Input: part model. Units: mm. Frame: model coordinates. A direction names the side the tool comes from. Coordinates: 2 decimals unless noted, no trailing zeros. Loops run counter-clockwise (first coordinate to the right, second up) from the corner with the lowest first, then second, coordinate; pieces in that order, holes last. Notation, with made-up numbers: M 80,40 L 119,40 A17 cw 119,71 Z; hole C -16.5,4.5 d10. An arc over 180 degrees is marked long. Use a Markdown table: item, result. Add a question column.
1. Section D-D on x = -46.5. Output: boundary loops of the cut face in (y, z), then the cut area to 3 significant figures.
2. Section A-A on x = -162.5. Output: boundary loops of the cut face in (y, z), then the cut area to 3 significant figures.
3. Pin query (flat end, axial travel): pin 1 (7 mm diameter, centred on x = -4.5, z = -101.5, fed in from -Y); pin 2 (8 mm diameter, centred on y = -15.5, z = -5.5, fed in from -X); pin 3 (6.5 mm diameter, centred on y = 6, z = 14, fed in from +X). Return the tip coordinate at first contact, or that it passes through.
4. Section B-B on z = -67. Output: boundary loops of the cut face in (x, y).
5. Section C-C on x = 70.5. Output: boundary loops of the cut face in (y, z), then the cut area to 3 significant figures.
6. Set-up query: faces 1 (the flat face through (-12, 12, -93)), 2 (the flat face through (159, 10, 10)), 3 (the flat face through (-157, -35, -8)), 4 (the flat face through (154, 0, 0)). Return all of +Z, -Z, +X, -X, +Y, -Y with unobstructed straight access to the full face (end or side cutting, diameter ignored); none if empty.
7. Draft query along Z for faces 5 (the flat face through (-159, 10, 10)), 6 (the flat face through (16, 10, -96)), 7 (the flat face through (0, 30, -86)), 8 (the flat face through (181, 10, 5)). Return one class per face: +Z half, -Z half, draft (parallel to the pull), parting line (faces both ways), or undercut.
8. Line query: L1, parallel to X at y = 31.2, z = -86; L2, parallel to X at y = 15, z = -3.5; L3, parallel to Z at x = 0, y = 33. Output: solid intervals per line, ascending. Write a range as [from, to].
```python
from build123d import *

# Parameters (mm, degrees)
EXTRUDE_1_DEPTH           = 20
SKETCH_18_W               = 10
SKETCH_18_H               = 10
CUT_EXTRUDE_6_DEPTH       = 10
SKETCH_20_W               = 40
SKETCH_20_H               = 4
EXTRUDE_5_DEPTH           = 10
SKETCH_8_W                = 4
SKETCH_8_H                = 32
SKETCH_25_W               = 246.903686524
SKETCH_25_H               = 75.06139437
CUT_EXTRUDE_7_DEPTH       = 30
SKETCH_11_W               = 4
SKETCH_11_H               = 32
SKETCH_26_W               = 20
SKETCH_26_H               = 20
EXTRUDE_6_DEPTH           = 70
SKETCH_28_W               = 20
SKETCH_28_H               = 20
EXTRUDE_7_DEPTH           = 70
SKETCH_29_W               = 26
SKETCH_29_H               = 10
CUT_EXTRUDE_8_DEPTH       = 20
SKETCH_31_R               = 10
CUT_EXTRUDE_10_DEPTH      = 101
SKETCH_32_R               = 10
EXTRUDE_8_DEPTH           = 8
CUT_EXTRUDE_11_DEPTH      = 95
EXTRUDE_9_DEPTH           = 24
CUT_EXTRUDE_12_DEPTH      = 215
SKETCH_36_R               = 6
SKETCH_36_R_2             = 4
EXTRUDE_10_DEPTH          = 4
SKETCH_38_W               = 10.504176023
SKETCH_38_H               = 23.874283345
SKETCH_38_W_2             = 11.702143621
CUT_EXTRUDE_13_DEPTH      = 195
CUT_EXTRUDE_13_DEPTH_BACK = 195


with BuildPart() as part:
    # 草图2 → 凸台-拉伸1 (new body)
    with BuildSketch(Plane(origin=(0, 0, 0), x_dir=(1, 0, 0), z_dir=(0, 1, 0))):
        with BuildLine():
            Line((-40, 84), (40, 84))
            ThreePointArc((40, 84), (124, 0), (40, -84))
            Line((40, -84), (-40, -84))
            ThreePointArc((-40, -84), (-124, 0), (-40, 84))
        make_face()
        with BuildLine():
            Line((-40, 80), (40, 80))
            ThreePointArc((40, 80), (120, 0), (40, -80))
            Line((40, -80), (-40, -80))
            ThreePointArc((-40, -80), (-120, 0), (-40, 80))
        make_face(mode=Mode.SUBTRACT)
    extrude(amount=EXTRUDE_1_DEPTH)

    # 草图18 → 切除-拉伸6 (cut)
    with BuildSketch(Plane(origin=(0, 0, -84), x_dir=(-1, 0, 0), z_dir=(0, 0, -1))):
        with Locations((0, 10)):
            Rectangle(SKETCH_18_W, SKETCH_18_H)
    extrude(amount=-CUT_EXTRUDE_6_DEPTH, mode=Mode.SUBTRACT)

    # 草图20 → 凸台-拉伸5 (add)
    with BuildSketch(Plane(origin=(0, 20, 0), x_dir=(1, 0, 0), z_dir=(0, 1, 0))):
        with Locations((0, 82)):
            Rectangle(SKETCH_20_W, SKETCH_20_H)
    extrude(amount=EXTRUDE_5_DEPTH)

    # 扫描1: sweep along a path in 草图9
    with BuildLine(Plane.XY) as sweep_1_path:
        Line((-124, 20), (-124, 0))
        Line((-124, 0), (-155, -40))
    # 草图8 → 扫描1 (sweep)
    with BuildSketch(Plane(origin=(0, 20, 0), x_dir=(1, 0, 0), z_dir=(0, 1, 0))):
        with Locations((-122, 0)):
            Rectangle(SKETCH_8_W, SKETCH_8_H)
    sweep(path=sweep_1_path.line, transition=Transition.RIGHT)

    # 草图25 → 切除-拉伸7 (cut)
    with BuildSketch(Plane(origin=(0, 20, 0), x_dir=(1, 0, 0), z_dir=(0, 1, 0))):
        with Locations((0.98973075, -53.530697185)):
            Rectangle(SKETCH_25_W, SKETCH_25_H)
    extrude(amount=-CUT_EXTRUDE_7_DEPTH, mode=Mode.SUBTRACT)

    # 扫描2: sweep along a path in 草图27
    with BuildLine(Plane.XY) as sweep_2_path:
        Line((124, 20), (124, 0))
        Line((124, 0), (155, -40))
    # 草图11 → 扫描2 (sweep)
    with BuildSketch(Plane(origin=(0, 20, 0), x_dir=(1, 0, 0), z_dir=(0, 1, 0))):
        with Locations((122, 0)):
            Rectangle(SKETCH_11_W, SKETCH_11_H)
    sweep(path=sweep_2_path.line, transition=Transition.RIGHT)

    # 草图26 → 凸台-拉伸6 (add)
    with BuildSketch(Plane.ZY.offset(124)):
        with Locations((0, 10)):
            Rectangle(SKETCH_26_W, SKETCH_26_H)
    extrude(amount=EXTRUDE_6_DEPTH)

    # 草图28 → 凸台-拉伸7 (add)
    with BuildSketch(Plane(origin=(124, 0, 0), x_dir=(0, 0, -1), z_dir=(1, 0, 0))):
        with Locations((0, 10)):
            Rectangle(SKETCH_28_W, SKETCH_28_H)
    extrude(amount=EXTRUDE_7_DEPTH)

    # 草图29 → 切除-拉伸8 (cut)
    with BuildSketch(Plane(origin=(0, 20, 0), x_dir=(1, 0, 0), z_dir=(0, 1, 0))):
        with Locations((-181, 0)):
            Rectangle(SKETCH_29_W, SKETCH_29_H)
        with Locations((181, 0)):
            Rectangle(SKETCH_29_W, SKETCH_29_H)
    extrude(amount=-CUT_EXTRUDE_8_DEPTH, mode=Mode.SUBTRACT)

    # 草图31 → 切除-拉伸10 (cut, through all)
    with BuildSketch(Plane.XY.offset(16)):
        with Locations((-159.742490313, -36.324570007)):
            Circle(SKETCH_31_R)
        with Locations((159.742490313, -36.324570007)):
            Circle(SKETCH_31_R)
    extrude(amount=-CUT_EXTRUDE_10_DEPTH, mode=Mode.SUBTRACT)

    # 草图32 → 凸台-拉伸8 (add, symmetric)
    with BuildSketch(Plane.XY):
        with Locations((-159.742490313, -36.324570007)):
            Circle(SKETCH_32_R)
        with Locations((159.742490313, -36.324570007)):
            Circle(SKETCH_32_R)
    extrude(amount=EXTRUDE_8_DEPTH, both=True)

    # 草图33 → 切除-拉伸11 (cut, through all)
    with BuildSketch(Plane.XY.offset(10)):
        with BuildLine():
            Line((-184, 20), (-199.388740024, 20))
            Line((-199.388740024, 20), (-199.388740024, 0))
            Line((-199.388740024, 0), (-184, 0))
            ThreePointArc((-184, 0), (-194, 10), (-184, 20))
        make_face()
        with BuildLine():
            Line((184, 20), (198.413524526, 20))
            Line((198.413524526, 20), (198.413524526, 0))
            Line((198.413524526, 0), (184, 0))
            ThreePointArc((184, 0), (194, 10), (184, 20))
        make_face()
    extrude(amount=-CUT_EXTRUDE_11_DEPTH, mode=Mode.SUBTRACT)

    # 草图34 → 凸台-拉伸9 (add)
    with BuildSketch(Plane(origin=(0, 0, -84), x_dir=(-1, 0, 0), z_dir=(0, 0, -1))):
        Polygon((20, 30), (-20, 30), (-20, 20), (-20, 0), (-12, 0), (-12, 20), (12, 20), (12, 0), (20, 0), (20, 20), align=None)
    extrude(amount=EXTRUDE_9_DEPTH)

    # 草图35 → 切除-拉伸12 (cut, through all)
    with BuildSketch(Plane(origin=(20, 0, 0), x_dir=(0, 0, -1), z_dir=(1, 0, 0))):
        Polygon((108, 20), (84, 0), (110.80524342, 0), align=None)
    extrude(amount=-CUT_EXTRUDE_12_DEPTH, mode=Mode.SUBTRACT)

    # 草图36 → 凸台-拉伸10 (add)
    with BuildSketch(Plane(origin=(0, 30, 0), x_dir=(1, 0, 0), z_dir=(0, 1, 0))):
        with Locations((0, 86)):
            Circle(SKETCH_36_R)
        with Locations((0, 86)):
            Circle(SKETCH_36_R_2, mode=Mode.SUBTRACT)
    extrude(amount=EXTRUDE_10_DEPTH)

    # 草图38 → 切除-拉伸13 (cut, two sides)
    with BuildSketch(Plane(origin=(0, 0, 0), x_dir=(0, 0, -1), z_dir=(1, 0, 0))) as cut_extrude_13_sk:
        with Locations((-13.252088011, -34.387428335)):
            Rectangle(SKETCH_38_W, SKETCH_38_H)
        with Locations((13.851071811, -34.387428335)):
            Rectangle(SKETCH_38_W_2, SKETCH_38_H)
    extrude(amount=CUT_EXTRUDE_13_DEPTH, mode=Mode.SUBTRACT)
    extrude(cut_extrude_13_sk.sketch, amount=-CUT_EXTRUDE_13_DEPTH_BACK, mode=Mode.SUBTRACT)


solid = part.part
```
Answers below:
| question | item | result |
|---|---|---|
| 1 | outline | M 0,-83.75 L 20,-83.75 L 20,-79.74 L 0,-79.74 Z |
| 1 | area | 80.3 mm² |
| 2 | outline | M -45.94,-8 L -26.71,-8 L -26.71,8 L -45.94,8 Z; M 0,-10 L 20,-10 L 20,10 L 0,10 Z |
| 2 | area | 708 mm² |
| 3 | pin 1 | stops at y = 20 |
| 3 | pin 2 | stops at x = -139.11 |
| 3 | pin 3 | stops at x = 124 |
| 4 | outline | M -90.67,0 L -83.71,0 L -83.71,20 L -90.67,20 Z; M 83.71,0 L 90.67,0 L 90.67,20 L 83.71,20 Z |
| 5 | outline | M 0,-78.27 L 20,-78.27 L 20,-73.96 L 0,-73.96 Z |
| 5 | area | 86.2 mm² |
| 6 | face 1 | -Z, -Y |
| 6 | face 2 | +Z, +X, +Y |
| 6 | face 3 | -Z, +X, -X, -Y |
| 6 | face 4 | +Z, -Z, +X |
| 7 | face 5 | +Z half |
| 7 | face 6 | -Z half |
| 7 | face 7 | undercut |
| 7 | face 8 | undercut |
| 8 | L1 | x = [-6, -4], [4, 6] |
| 8 | L2 | x = [-168, -119.92], [119.92, 168] |
| 8 | L3 | z = [-92, -90], [-82, -80] |
